from build123d import *

# Parameters (mm, degrees)
BOSS_EXTRUDE1_DEPTH = 63.5
BOSS_EXTRUDE2_DEPTH = 63.5
SKETCH6_R           = 9.525
CUT_EXTRUDE1_DEPTH  = 20.05


with BuildPart() as part:
    # Sketch3 → Boss-Extrude1 (new body)
    with BuildSketch(Plane(origin=(0, 0, 0), x_dir=(1, 0, 0), z_dir=(0, 1, 0))):
        Polygon((0, 0), (63.5, 0), (63.5, 19.05), (19.05, 19.05), (19.05, 63.5), (0, 63.5), align=None)
    extrude(amount=BOSS_EXTRUDE1_DEPTH)

    # Sketch5 → Boss-Extrude2 (add)
    with BuildSketch(Plane(origin=(63.5, 0, 0), x_dir=(0, 0, -1), z_dir=(1, 0, 0))):
        Polygon((0, 63.5), (-63.5, 63.5), (-63.5, 0), (-44.45, 0), (-44.45, 44.45), (0, 44.45), align=None)
    extrude(amount=-BOSS_EXTRUDE2_DEPTH)

    # Sketch6 → Cut-Extrude1 (cut, through all)
    with BuildSketch(Plane(origin=(19.05, 0, 0), x_dir=(0, 0, -1), z_dir=(1, 0, 0))):
        with Locations((44.45, 31.75)):
            Circle(SKETCH6_R)
    extrude(amount=-CUT_EXTRUDE1_DEPTH, mode=Mode.SUBTRACT)


solid = part.part
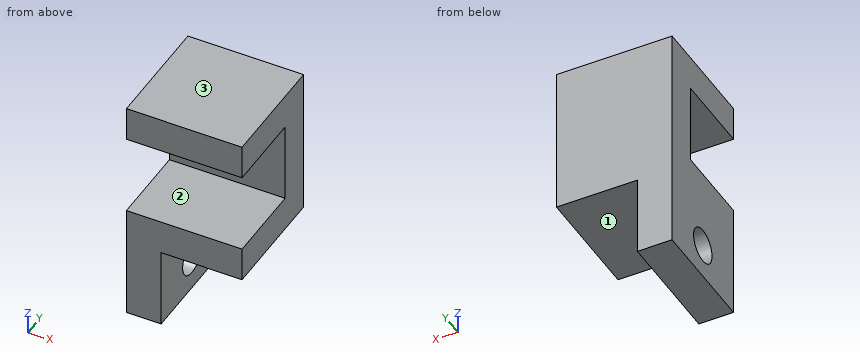
Model file for the job. Use its own axes, mm. Face numbers are marked on the shaded views. A direction names the side the tool comes from. Coordinates: 2 decimals unless noted, no trailing zeros. Write each loop counter-clockwise with the first axis right and the second up, starting at its lowest first coordinate (ties: lowest second). Pieces come first, ordered by that corner, then holes. Notation, with made-up numbers: (-24.5, 35.5) - (15.5, 35.5) arc R19 cw to (15.5, 53.5) - close; hole circle Ø6 at (-14.5, 29.5). An arc over 180 degrees is marked (long way). Write each question's results on one line, items separated by ' | '. Start each with the question number.
1) Cut at A-A (y = 31.75). Write the cut outline in (x, z) (3 decimals).
2) Cut at D-D (x = 57). Write the cut outline in (y, z).
3) Flat gauge pins, fed straight in: P1, Ø5, axis at x = 8.5, z = -13.5, coming from the -Y side; P2, Ø13.5, axis at x = 40.5, y = 23.5, coming from the -Z side. Where does each tip first touch, or does it go through?
4) 3-axis set-ups, long thin cutter, end or side, ignore diameter. For the marked faces 1, 2 and 3: which of +Z, -Z, +X, -X, +Y, -Y reach the whole face in a straight line?
5) Probe line 1 along Z through (x, y) = (10, 32); line 2 along Z through (x, y) = (7, 31); line 3 along Z through (x, y) = (26, 13.5). List the from-to ranges inside material, lowest first. Write a range as from..to.
6) Cut at C-C (y = 12.5). Write the cut outline in (x, z).
7) Cut at B-B (z = -44.45). Write the cut outline in (x, y) (3 decimals), then the cut area to 3 significant figures.
Returned:
1) outline: (0, -63.5) - (19.05, -63.5) - (19.05, -53.975) - (0, -53.975) - close; (0, -34.925) - (19.05, -34.925) - (19.05, -19.05) - (63.5, -19.05) - (63.5, 0) - (0, 0) - close; (0, 44.45) - (63.5, 44.45) - (63.5, 63.5) - (0, 63.5) - close
2) outline: (0, -19.05) - (63.5, -19.05) - (63.5, 63.5) - (0, 63.5) - (0, 44.45) - (44.45, 44.45) - (44.45, 0) - (0, 0) - close
3) P1: y = 0 | P2: z = -19.05
4) face 1: -Z, +X, +Y, -Y | face 2: +X, -X, -Y | face 3: +Z, +X, -X, +Y, -Y
5) line 1: -63.5..-53.97, -34.93..0, 44.45..63.5 | line 2: -63.5..-53.95, -34.95..0, 44.45..63.5 | line 3: -19.05..0, 44.45..63.5
6) outline: (0, -63.5) - (19.05, -63.5) - (19.05, -19.05) - (63.5, -19.05) - (63.5, 0) - (0, 0) - close; (0, 44.45) - (63.5, 44.45) - (63.5, 63.5) - (0, 63.5) - close
7) outline: (0, 0) - (19.05, 0) - (19.05, 22.225) - (0, 22.225) - close; (0, 41.275) - (19.05, 41.275) - (19.05, 63.5) - (0, 63.5) - close | area: 847 mm^2
